Part print with two shaded views. Sizes in mm from the minimum x, y, z corner. Give positions to 0.01 mm unless a question says otherwise; leave off trailing zeros. Write each loop counter-clockwise with the first axis right and the second up, starting at its lowest first coordinate (ties: lowest second). Pieces come first, ordered by that corner, then holes.
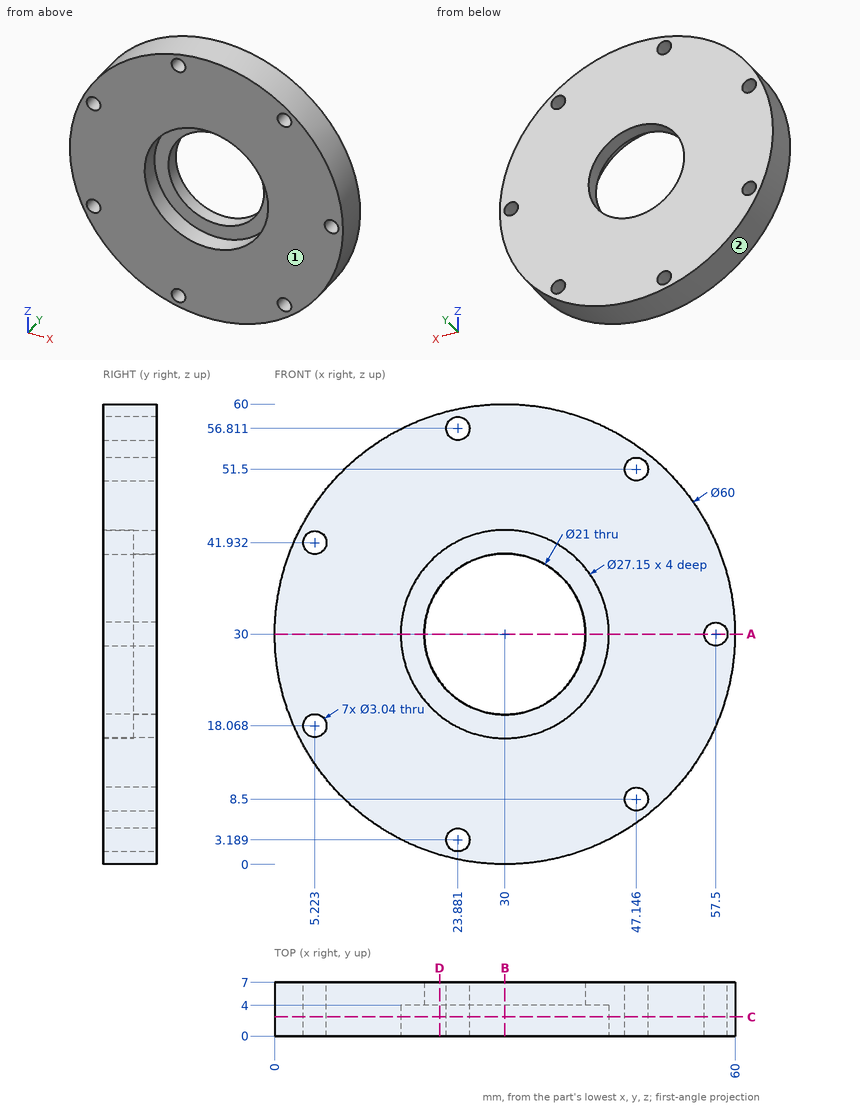
1) Saw through at C-C (y = 2.5). State how many separate pieces and enclosed holes the cut face has, and give its area (3 significant figures).
Check result:
separate pieces: 1
enclosed holes: 8
area: 2,200 mm2
2) Drill centre lines: L1, parallel to X at y = 3, z = 30 (1 decimal); L2, parallel to X at y = 4.25, z = 30; L3, parallel to Y at x = 39, z = 38.5. Where is each one in solid material? Low to high.
Check result:
L1: x = 0 to 16.4, 43.6 to 56, 59 to 60
L2: x = 0 to 19.5, 40.5 to 55.98, 59.02 to 60
L3: y = 4 to 7
3) Saw through at A-A (z = 30). Write the cut outline in (x, y) (1 decimal), and give its area (3 significant figures).
Check result:
outline: (0, 0) - (16.4, 0) - (16.4, 4) - (19.5, 4) - (19.5, 7) - (0, 7) - close; (40.5, 4) - (43.6, 4) - (43.6, 0) - (56, 0) - (56, 7) - (40.5, 7) - close; (59, 0) - (60, 0) - (60, 7) - (59, 7) - close
area: 227 mm2
4) Saw through at B-B (x = 30). Write the cut outline in (y, z) (1 decimal).
Check result:
outline: (0, 0) - (7, 0) - (7, 19.5) - (4, 19.5) - (4, 16.4) - (0, 16.4) - close; (0, 43.6) - (4, 43.6) - (4, 40.5) - (7, 40.5) - (7, 60) - (0, 60) - close
5) Saw through at D-D (x = 21.5). Write the cut outline in (y, z) (1 decimal), and give its area (3 significant figures).
Check result:
outline: (0, 1.2) - (7, 1.2) - (7, 23.8) - (4, 23.8) - (4, 19.4) - (0, 19.4) - close; (0, 40.6) - (4, 40.6) - (4, 36.2) - (7, 36.2) - (7, 58.8) - (0, 58.8) - close
area: 281 mm2
6) Mould opens along X. For the marked faces 1 and 2 say: +X half, -X half, draft (parallel to the pull), parting line (faces both ways), or undercut.
Check result:
face 1: draft
face 2: parting line
7) Flat gauge pins, fed straight in: P1, Ø2, axis at x = 26.5, y = 4, coming from the -Z side; P2, Ø10, axis at x = 20.5, z = 12.5, coming from the -Y side; P3, Ø2, axis at y = 2.5, z = 18.5, coming from the -X side; P4, Ø1.5, axis at x = 35.5, y = 4, coming from the -Z side. Where does each tip first touch, or does it go through?
Check result:
P1: stops at z = 0.1
P2: stops at y = 0
P3: stops at x = 1.9
P4: stops at z = 0.38
